Design review of the part built by this model. Coordinates are the model's own, in mm. Round coordinates to 2 decimals unless told otherwise and drop trailing zeros.
from build123d import *

# Parameters (mm, degrees)
SKETCH1_W               = 406.4
SKETCH1_H               = 508
BOSS_EXTRUDE1_DEPTH     = 3.175
SKETCH2_R               = 14.2875
CUT_EXTRUDE1_DEPTH      = 3.175
SKETCH3_R               = 2.4892
CUT_EXTRUDE2_DEPTH      = 1
CUT_EXTRUDE2_DEPTH_BACK = 4.175
SKETCH4_R               = 2.0193
CUT_EXTRUDE3_DEPTH      = 1
CUT_EXTRUDE3_DEPTH_BACK = 4.175


with BuildPart() as part:
    # Sketch1 → Boss-Extrude1 (new body)
    with BuildSketch(Plane(origin=(0, 0, 0), x_dir=(1, 0, 0), z_dir=(0, 1, 0))):
        with Locations((203.2, 254)):
            Rectangle(SKETCH1_W, SKETCH1_H)
    extrude(amount=BOSS_EXTRUDE1_DEPTH)

    # Sketch2 → Cut-Extrude1 (cut)
    with BuildSketch(Plane(origin=(0, 3.175, 0), x_dir=(1, 0, 0), z_dir=(0, 1, 0))):
        with Locations((50.8, 419.1)):
            Circle(SKETCH2_R)
        with Locations((165.1, 419.1)):
            Circle(SKETCH2_R)
        with Locations((50.8, 88.9)):
            Circle(SKETCH2_R)
        with Locations((165.1, 88.9)):
            Circle(SKETCH2_R)
    extrude(amount=-CUT_EXTRUDE1_DEPTH, mode=Mode.SUBTRACT)

    # Sketch3 → Cut-Extrude2 (cut, two sides)
    with BuildSketch(Plane(origin=(0, 3.175, 0), x_dir=(1, 0, 0), z_dir=(0, 1, 0))) as cut_extrude2_sk:
        with Locations((38.1, 12.7)):
            Circle(SKETCH3_R)
        with Locations((63.5, 12.7)):
            Circle(SKETCH3_R)
        with Locations((127, 12.7)):
            Circle(SKETCH3_R)
        with Locations((152.4, 12.7)):
            Circle(SKETCH3_R)
        with Locations((177.8, 12.7)):
            Circle(SKETCH3_R)
        with Locations((203.2, 12.7)):
            Circle(SKETCH3_R)
        with Locations((228.6, 12.7)):
            Circle(SKETCH3_R)
        with Locations((254, 12.7)):
            Circle(SKETCH3_R)
        with Locations((279.4, 12.7)):
            Circle(SKETCH3_R)
        with Locations((304.8, 12.7)):
            Circle(SKETCH3_R)
        with Locations((330.2, 12.7)):
            Circle(SKETCH3_R)
        with Locations((355.6, 12.7)):
            Circle(SKETCH3_R)
        with Locations((381, 12.7)):
            Circle(SKETCH3_R)
        with Locations((381, 495.3)):
            Circle(SKETCH3_R)
        with Locations((355.6, 495.3)):
            Circle(SKETCH3_R)
        with Locations((330.2, 495.3)):
            Circle(SKETCH3_R)
        with Locations((304.8, 495.3)):
            Circle(SKETCH3_R)
        with Locations((279.4, 495.3)):
            Circle(SKETCH3_R)
        with Locations((254, 495.3)):
            Circle(SKETCH3_R)
        with Locations((228.6, 495.3)):
            Circle(SKETCH3_R)
        with Locations((203.2, 495.3)):
            Circle(SKETCH3_R)
        with Locations((177.8, 495.3)):
            Circle(SKETCH3_R)
        with Locations((152.4, 495.3)):
            Circle(SKETCH3_R)
        with Locations((127, 495.3)):
            Circle(SKETCH3_R)
        with Locations((63.5, 495.3)):
            Circle(SKETCH3_R)
        with Locations((38.1, 495.3)):
            Circle(SKETCH3_R)
        with Locations((101.6, 12.7)):
            Circle(SKETCH3_R)
    extrude(amount=CUT_EXTRUDE2_DEPTH, mode=Mode.SUBTRACT)
    extrude(cut_extrude2_sk.sketch, amount=-CUT_EXTRUDE2_DEPTH_BACK, mode=Mode.SUBTRACT)

    # Sketch4 → Cut-Extrude3 (cut, two sides)
    with BuildSketch(Plane(origin=(0, 3.175, 0), x_dir=(1, 0, 0), z_dir=(0, 1, 0))) as cut_extrude3_sk:
        with Locations((76.2, 419.1)):
            Circle(SKETCH4_R)
        with Locations((25.4, 419.1)):
            Circle(SKETCH4_R)
        with Locations((38.1, 441.097045256)):
            Circle(SKETCH4_R)
        with Locations((63.5, 441.097045256)):
            Circle(SKETCH4_R)
        with Locations((63.5, 397.102954744)):
            Circle(SKETCH4_R)
        with Locations((38.1, 397.102954744)):
            Circle(SKETCH4_R)
        with Locations((147.139487788, 437.060512212)):
            Circle(SKETCH4_R)
        with Locations((183.060512212, 437.060512212)):
            Circle(SKETCH4_R)
        with Locations((183.060512212, 401.139487788)):
            Circle(SKETCH4_R)
        with Locations((147.139487788, 401.139487788)):
            Circle(SKETCH4_R)
        with Locations((147.139487788, 106.860512212)):
            Circle(SKETCH4_R)
        with Locations((183.060512212, 106.860512212)):
            Circle(SKETCH4_R)
        with Locations((183.060512212, 70.939487788)):
            Circle(SKETCH4_R)
        with Locations((147.139487788, 70.939487788)):
            Circle(SKETCH4_R)
        with Locations((38.1, 110.897045256)):
            Circle(SKETCH4_R)
        with Locations((63.5, 110.897045256)):
            Circle(SKETCH4_R)
        with Locations((63.5, 66.902954744)):
            Circle(SKETCH4_R)
        with Locations((38.1, 66.902954744)):
            Circle(SKETCH4_R)
        with Locations((25.4, 88.9)):
            Circle(SKETCH4_R)
        with Locations((76.2, 88.9)):
            Circle(SKETCH4_R)
    extrude(amount=CUT_EXTRUDE3_DEPTH, mode=Mode.SUBTRACT)
    extrude(cut_extrude3_sk.sketch, amount=-CUT_EXTRUDE3_DEPTH_BACK, mode=Mode.SUBTRACT)


solid = part.part
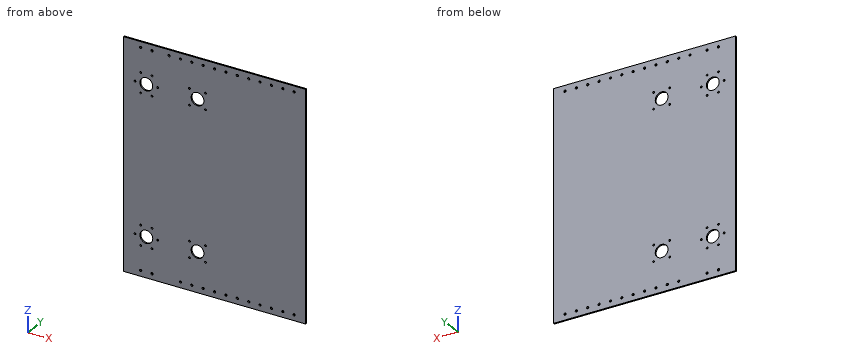
1) Take a section at A-A on y = 1.5. State how many separate pieces and enclosed holes the cut face has, plus the area to 3 significant figures.
Results:
separate pieces: 1
enclosed holes: 51
area: 203,000 mm2
2) To check wall thickness, follow line 1 along X through (y, z) = (2.1, -88.9); line 2 along Z through (x, y) = (331, 0.7). State the ranges of each line that lie inside material, in increasing order.
Results:
line 1: x = 0 to 23.38, 27.42 to 36.51, 65.09 to 74.18, 78.22 to 150.81, 179.39 to 406.4
line 2: z = -508 to -497.66, -492.94 to -15.06, -10.34 to 0
3) Clearance check with a flat-ended pin moving along its axis: P1, Ø5.5, axis at x = 147.14, z = -401.14, coming from the -Y side. State where the tip first meets the part, or that it passes through.
Results:
P1: stops at y = 0
